```python
from build123d import *

# Parameters (mm, degrees)
F0_W     = 15.7734
F0_H     = 7.7724
F1_DEPTH = 9.5504
F3_W     = 12.7254
F3_H     = 4.7244
F3_R     = 1.524
F4_DEPTH = 8.0772
F5_R     = 2.4384
F6_DEPTH = 1.8288


with BuildPart() as f1:
    # F0 (on Top) → F1 (new body)
    with BuildSketch(Plane.XY):
        Rectangle(F0_W, F0_H)
    extrude(amount=F1_DEPTH)

    # F3 (on face) → F4 (cut)
    with BuildSketch(Plane.XY.offset(9.5504)):
        Rectangle(F3_W, F3_H)
        Circle(F3_R, mode=Mode.SUBTRACT)
    extrude(amount=-F4_DEPTH, mode=Mode.SUBTRACT)

    # F5 (on face) → F6 (join)
    with BuildSketch(Plane(origin=(0, 0, 0), x_dir=(1, 0, 0), z_dir=(0, 0, -1))):
        with Locations((-3.8989, 0)):
            Circle(F5_R)
        with Locations((4.0005, 0)):
            Circle(F5_R)
    extrude(amount=F6_DEPTH)


solid = f1.part
```
Source: CAD feature listing. Evaluate the final solid. Frame: model axes, mm. A direction names the side the tool comes from. Give positions to 0.01 mm unless a question says otherwise; leave off trailing zeros. Write each loop counter-clockwise with the first axis right and the second up, starting at its lowest first coordinate (ties: lowest second). Pieces come first, ordered by that corner, then holes.
1. Material intervals for line 1 along X through (y, z) = (-2, 1.75); line 2 along Y through (x, z) = (-5, 8.5); line 3 along Y through (x, z) = (-0.5, 2.5), sorted ascending.
2. Pull-direction query (X, two-part tool) for faces 4 (the face through (6.363, 0, 6)), 5 (the face through (0, -3.886, 5)), 6 (the face through (-0.2, 1.51, 5.57)), 7 (the face through (-7.887, 0, 5)); classes: +X half, -X half, draft (parallel to the pull), parting line (faces both ways), or undercut.
3. Section query B-B (y = 0). Return the cut outline in (x, z), then the cut area to 3 significant figures.
4. Access query for faces 1 (the face through (0, -2.362, 6)), 2 (the face through (0, 0, 0)), 3 (the face through (4, 0, -1.829)). Directions: +Z, -Z, +X, -X, +Y, -Y. A direction counts if a zero-diameter tool reaches every point of the face in a straight line with its end or side. Return the directions, or none.
5. Section query D-D (y = 1.25). Return the cut outline in (x, z).
6. Section query C-C (x = 0). Return the cut outline in (y, z).
7. Section query A-A (z = 5.5). Return the cut outline in (x, y).
Output values:
1. line 1: x = -7.89 to -6.36, 6.36 to 7.89
1. line 2: y = -3.89 to -2.36, 2.36 to 3.89
1. line 3: y = -3.89 to -2.36, -1.44 to 1.44, 2.36 to 3.89
2. face 4: undercut
2. face 5: draft
2. face 6: undercut
2. face 7: -X half
3. outline: (-7.89, 0) - (-6.34, 0) - (-6.34, -1.83) - (-1.46, -1.83) - (-1.46, 0) - (1.56, 0) - (1.56, -1.83) - (6.44, -1.83) - (6.44, 0) - (7.89, 0) - (7.89, 9.55) - (6.36, 9.55) - (6.36, 1.47) - (1.52, 1.47) - (1.52, 9.55) - (-1.52, 9.55) - (-1.52, 1.47) - (-6.36, 1.47) - (-6.36, 9.55) - (-7.89, 9.55) - close
3. area: 90.3 mm2
4. face 1: +Z
4. face 2: -Z
4. face 3: -Z, +X, -X, +Y, -Y
5. outline: (-7.89, 0) - (-5.99, 0) - (-5.99, -1.83) - (-1.81, -1.83) - (-1.81, 0) - (1.91, 0) - (1.91, -1.83) - (6.09, -1.83) - (6.09, 0) - (7.89, 0) - (7.89, 9.55) - (6.36, 9.55) - (6.36, 1.47) - (0.87, 1.47) - (0.87, 9.55) - (-0.87, 9.55) - (-0.87, 1.47) - (-6.36, 1.47) - (-6.36, 9.55) - (-7.89, 9.55) - close
6. outline: (-3.89, 0) - (3.89, 0) - (3.89, 9.55) - (2.36, 9.55) - (2.36, 1.47) - (1.52, 1.47) - (1.52, 9.55) - (-1.52, 9.55) - (-1.52, 1.47) - (-2.36, 1.47) - (-2.36, 9.55) - (-3.89, 9.55) - close
7. outline: (-7.89, -3.89) - (7.89, -3.89) - (7.89, 3.89) - (-7.89, 3.89) - close; circle Ø3.05 at (0, 0); hole (-6.36, -2.36) - (6.36, -2.36) - (6.36, 2.36) - (-6.36, 2.36) - close
